Autodesk Inventor part; units mm, degrees
ref_plane "YZ Plane" through (0, 0, 0) normal (1, 0, 0) x (0, 1, 0)
ref_plane "XZ Plane" through (0, 0, 0) normal (0, 1, 0) x (-1, 0, 0)
ref_plane "XY Plane" through (0, 0, 0) normal (0, 0, 1) x (1, 0, 0)
sketch "Skizze3" plane through (0, 0, 0) normal (0, 0, 1) x (1, 0, 0)
  line L0 (-225, 400) -> (225, 400)
  line L1 (225, 400) -> (225, -400)
  line L2 (225, -400) -> (-225, -400)
  line L3 (-225, -400) -> (-225, 400)
  arc A0 (-195.1149, 0) -> (-225, -400) centre (2466.8593, -400) ccw
  arc A1 (-195.1149, 0) -> (-195, 270) centre (-1096.0822, 135.3833) ccw
  arc A2 (225, -400) -> (191.0498, 0) centre (-2148.3658, -400) ccw
  arc A3 (195, 400) -> (191.0498, 0) centre (1296.9948, 189.0977) ccw
  arc A4 (195, 400) -> (-98.428, 330) centre (195, -250) ccw
  arc A5 (-112.8051, 0) -> (-95, -400) centre (880.9564, -156.1612) ccw
  arc A6 (-112.8051, 0) -> (-145, 340) centre (-793.9104, 107.0299) ccw
  arc A7 (-135, 310) -> (-195, 270) centre (195, -250) ccw
  arc A8 (-65, 0) -> (-5, -400) centre (1298.3333, 0) ccw
  arc A9 (-98.428, 330) -> (-135, 310) centre (195, -250) ccw construction
  line L4 (-65, 0) -> (-65, 238.5671) construction
  arc A10 (-65, 142.5015) -> (-115, 370) centre (-607.5556, 142.5015) ccw
  line L5 (-65, 142.5015) -> (-65, 0)
  arc A11 (-115, 370) -> (-145, 340) centre (-60.8986, 285.8986) ccw
  arc A12 (-98.428, 330) -> (-225, 400) centre (-144761.9711, -261097.0223) ccw construction
  arc A13 (175.6814, 150) -> (-98.428, 330) centre (-1149.0878, -1568.6875) ccw construction
  point P0 (0, 0)
  point P1 (-225.0722, 0)
  point P2 (0, 400.05)
  point P3 (-225, 0)
  point P4 (0, 400)
  dimension "d5" = 800
  dimension "d8" = 450
  dimension "d9" = 670
  dimension "d10" = 30
  dimension "d11" = 40
  dimension "d12" = 30
  dimension "d14" = 50
  dimension "d16" = 130
  dimension "d18" = 90
  dimension "d19" = 740
  dimension "d21" = 90
  dimension "d22" = 230
  dimension "d23" = 140
  dimension "d26" = 100
  dimension "d28" = 730
  dimension "d34" = 160
  dimension "d35" = 30
  dimension "d36" = 770
  dimension "d38" = 100
  dimension "d51" = 323.428
  dimension "d52" = 250
  dimension "d53" = 2170
extrude "Extrusion3" add sketch "Skizze3" against normal blind 150 contours A10 L5 A8 L2 A5 A6 A11
fillet "Rundung1" radius 10 8 edges at (-65, 71.2508, 0) (-49.9166, -202.2375, 0) (-106.3148, 350.1654, 0) (-73.4224, 237.729, 0) (-124.0049, -200.8948, 0) (-106.2073, 156.2669, 0) (-139.828, 325.0573, 0) (-131.6093, 356.6093, 0)
sketch "Skizze8" plane through (-95, -400, -150) normal (0, -1, 0) x (1, 0, 0)
  line L0 (0, 140) -> (0, 0)
  line L1 (90, 0) -> (0, 0)
  circle A0 centre (30, 70) radius 12.5
  point P0 (95, 150)
  dimension "d62" = 25
  dimension "d63" = 70
  dimension "d64" = 30
extrude "Extrusion4" cut sketch "Skizze8" against normal blind 100
properties part number "UA-70 Denkmal2"
For this review, take the finished solid that the model builds, in its own axes (mm). A direction names the side the tool comes from. Round coordinates to 2 decimals unless told otherwise and drop trailing zeros. Loops run counter-clockwise (first coordinate to the right, second up) from the corner with the lowest first, then second, coordinate; pieces in that order, holes last. Notation, with made-up numbers: (33, 53.5) - (68, 53.5) arc R20 cw to (68, 92.5) - close; hole circle Ø11 at (-39, 61.25). An arc over 180 degrees is marked (long way). One line per item, written item: value. Start each with the question number.
Item 1: For L1, parallel to Z at x = -65, y = -346; L2, parallel to Z at x = -112, y = -27.5; L3, parallel to X at y = 311.5, z = -29.5, list the stretches that pass through material, from the lowest coordinate up.
Item 2: For faces 5 (the flat face through (-65, 72, -79)), 6 (the cylindrical face through (-66.627, -350.7, -67.606)), 7 (the flat face through (-92, -105, 0)), list the 3-axis set-ups (+Z, -Z, +X, -X, +Y, -Y) from which the entire face can be reached by the end or side of a thin tool; tool diameter is ignored.
Item 3: Take a section at B-B (z = -23). Give the boundary of the cut face in (x, y).
Item 4: Take a section at A-A (z = -80). Give the boundary of the cut face in (x, y).
Item 5: The part is to be moulded in two halves that separate along Y. For faces 1 (the flat face through (-65, -300, -80)), 2 (the cylindrical face through (-131.4, 356.82, -79.02)), 3 (the cylindrical face through (-124.126, -198.076, -79.02)), 4 (the cylindrical face through (-107.294, 169.62, -79.02)), say which applies: +Y half, -Y half, draft (parallel to the pull), parting line (faces both ways), or undercut.
Item 6: Clearance check with flat-ended pins moving along their axes: pin 1 Ø1.5 at (y, z) = (-218.5, -22.5) entering from +X; pin 2 Ø3 at (y, z) = (-254.5, -43) entering from -X. State where each tip first meets the part, or that it passes through.
Answer below:
1. L1: z = -150 to -92.5, -67.5 to 0
1. L2: z = -150 to -1.52
1. L3: x = -135.46 to -91.99
2. face 5: +Z, -Z, +X, +Y
2. face 6: -Y
2. face 7: +Z, +X, -X, +Y, -Y
3. outline: (-145, 340) arc R689.46 cw to (-112.81, 0) arc R1005.96 ccw to (-95, -400) - (-5, -400) arc R1363.33 cw to (-65, 0) - (-65, 142.5) arc R542.56 ccw to (-115, 370) arc R100 ccw to start
4. outline: (-145, 340) arc R689.46 cw to (-112.81, 0) arc R1005.96 ccw to (-95, -400) - (-77.5, -400) - (-77.5, -300) - (-52.5, -300) - (-52.5, -400) - (-5, -400) arc R1363.33 cw to (-65, 0) - (-65, 142.5) arc R542.56 ccw to (-115, 370) arc R100 ccw to start
5. face 1: -Y half
5. face 2: +Y half
5. face 3: undercut
5. face 4: undercut
6. pin 1: stops at x = -47.25
6. pin 2: stops at x = -120.33
